Autodesk Inventor part; units mm, degrees
ref_plane "YZ Plane" through (0, 0, 0) normal (1, 0, 0) x (0, 1, 0)
ref_plane "XZ Plane" through (0, 0, 0) normal (0, 1, 0) x (-1, 0, 0)
ref_plane "XY Plane" through (0, 0, 0) normal (0, 0, 1) x (1, 0, 0)
sketch "Sketch1" plane through (0, 0, 0) normal (0, 1, 0) x (-1, 0, 0)
  line L0 (20, 0) -> (89.97, 0)
  line L1 (109.97, -20) -> (109.97, -60)
  line L2 (89.97, -80) -> (20, -80)
  line L3 (0, -60) -> (0, -20)
  line L4 (79.7968, -72.5282) -> (60, -72.5282)
  line L5 (60, -72.5282) -> (60, -75.5)
  line L6 (60, -75.5) -> (79.7968, -75.5)
  line L7 (79.7968, -75.5) -> (79.7968, -72.5282)
  circle A0 centre (101.97, -32.634) radius 1.143
  circle A1 centre (101.97, -47.366) radius 1.143
  circle A2 centre (8, -32.634) radius 1.143
  circle A3 centre (8, -47.366) radius 1.143
  arc A4 (109.97, -20) -> (89.97, 0) centre (89.97, -20) ccw
  arc A5 (0, -60) -> (20, -80) centre (20, -60) ccw
  arc A6 (89.97, -80) -> (109.97, -60) centre (89.97, -60) ccw
  arc A7 (20, 0) -> (0, -20) centre (20, -20) ccw
  line L8 (49.7968, -4.5) -> (30, -4.5)
  line L9 (30, -4.5) -> (30, -7.4718)
  line L10 (30, -7.4718) -> (49.7968, -7.4718)
  line L11 (49.7968, -7.4718) -> (49.7968, -4.5)
  line L12 (49.7968, -72.5282) -> (30, -72.5282)
  line L13 (30, -72.5282) -> (30, -75.5)
  line L14 (30, -75.5) -> (49.7968, -75.5)
  line L15 (49.7968, -75.5) -> (49.7968, -72.5282)
  line L16 (60, -7.4718) -> (79.7968, -7.4718)
  line L17 (79.7968, -7.4718) -> (79.7968, -4.5)
  line L18 (79.7968, -4.5) -> (60, -4.5)
  line L19 (60, -4.5) -> (60, -7.4718)
  point P0 (0, 0)
  point P1 (109.97, -80)
  point P2 (109.97, 0)
  point P3 (0, -80)
  dimension "d0" = 109.97
  dimension "d1" = 80
  dimension "d2" = 19.7968
  dimension "d3" = 2.9718
  dimension "d7" = 4.5
  dimension "d9" = 2.286
  dimension "d10" = 2.286
  dimension "d11" = 14.732
  dimension "d12" = 32.634
  dimension "d13" = 8
  dimension "d14" = 8
  dimension "d15" = 2.286
  dimension "d16" = 2.286
  dimension "d17" = 8
  dimension "d18" = 8
  dimension "d19" = 20
  dimension "d20" = 20
  dimension "d21" = 20
  dimension "d24" = 19.7968
  dimension "d25" = 30
  dimension "d30" = 2.9718
  dimension "d33" = 4.5
  dimension "d34" = 10.2032
  dimension "d35" = 32.634
  dimension "d36" = 14.732
extrude "Extrusion4" add sketch "Sketch1" along normal blind 3.175
equation "\"d10\" = d9"
equation "\"d12\" = -0.5 * d11 + 0.5 * d1"
equation "\"d15\" = d9"
equation "\"d16\" = d9"
equation "\"d24\" = d2"
equation "\"d30\" = d3"
equation "\"d35\" = d12"
equation "\"d36\" = d11"
properties part number "base_plate"
Check sheet for the modelled part. Datum: model origin and axes. Units: mm. A direction names the side the tool comes from. Coordinates: 2 decimals unless noted, no trailing zeros. Write each loop counter-clockwise with the first axis right and the second up, starting at its lowest first coordinate (ties: lowest second). Pieces come first, ordered by that corner, then holes. Notation, with made-up numbers: M 66,65 L 73,65 A18 ccw 73,98 Z; hole C 81.5,48.25 d9. An arc over 180 degrees is marked long. Write item = value, one per line. Start each with the question number.
1. Sectioned sample at A-A (x = -101.97). Record the cut outline in (y, z) (3 decimals), then the cut area to 3 significant figures.
2. Mould release check, pull along X, two halves, no side actions. Record for faces 3 (the cylindrical face through (-103.956, 1.565, -5.703)), 4 (the flat face through (-40, 2, -75.5)), 5 (the flat face through (-55, 2, -80)): pulls with the +X half, pulls with the -X half, needs draft (parallel to the pull), parting line crosses it, or undercut.
3. Sectioned sample at C-C (x = -65). Record the cut outline in (y, z) (3 decimals).
4. Thickness scan on probe 1 along Z at (x, y) = (-39.5, 2.05); probe 2 along X at (y, z) = (1.7, -6); probe 3 along Z at (x, y) = (-8, 1.8). Record the ranges inside material, lowest first.
5. Go/stop test with flat-tipped pins: pin 1 (0.9 mm diameter, centred on y = 2.5, z = -74, fed in from +X); pin 2 (1.5 mm diameter, centred on y = 1, z = -6.5, fed in from -X); pin 3 (0.9 mm diameter, centred on y = 1.5, z = -74.5, fed in from +X). Record where each tip stops, or that it passes through.
6. Sectioned sample at B-B (y = 2.5). State how many separate pieces and enclosed holes the cut face has, then the cut area to 3 significant figures.
7. Sectioned sample at D-D (z = -10). Record the cut outline in (x, y) (1 decimal), then the cut area to 3 significant figures.
8. Tool access check on faces 1 (the flat face through (-70, 2, -4.5)), 2 (the cylindrical face through (-6.014, 1.565, -74.297)). Record the directions out of +Z, -Z, +X, -X, +Y, -Y that give a thin tool (end or side, any length) a straight path to the whole face; none if there is none.
The answers:
q1.outline = M 0,-76 L 3.175,-76 L 3.175,-48.509 L 0,-48.509 Z; M 0,-46.223 L 3.175,-46.223 L 3.175,-33.777 L 0,-33.777 Z; M 0,-31.491 L 3.175,-31.491 L 3.175,-4 L 0,-4 Z
q1.area = 214 mm²
q2.face_3 = pulls with the -X half
q2.face_4 = undercut
q2.face_5 = needs draft
q3.outline = M 0,-80 L 3.175,-80 L 3.175,-75.5 L 0,-75.5 Z; M 0,-72.528 L 3.175,-72.528 L 3.175,-7.472 L 0,-7.472 Z; M 0,-4.5 L 3.175,-4.5 L 3.175,0 L 0,0 Z
q4.probe_1 = -80 to -75.5, -72.53 to -7.47, -4.5 to 0
q4.probe_2 = -104.25 to -79.8, -60 to -49.8, -30 to -5.72
q4.probe_3 = -76 to -48.51, -46.22 to -33.78, -31.49 to -4
q5.pin_1 = -5.29
q5.pin_2 = -105.38
q5.pin_3 = -5.77
q6.separate_pieces = 1
q6.enclosed_holes = 8
q6.area = 8,200 mm²
q7.outline = M -107.3,0 L -2.7,0 L -2.7,3.2 L -107.3,3.2 Z
q7.area = 332 mm²
q8.face_1 = +Y, -Y
q8.face_2 = -Z, +X, +Y, -Y
